from build123d import *

# Parameters (mm, degrees)
SKETCH1_R           = 3.175
EXTRUSION2_DEPTH    = 6.35
SKETCH1_3_R         = 6.35
BOSS_EXTRUDE1_DEPTH = 6.35
SKETCH1_4_R         = 3.175
CUT_EXTRUDE1_DEPTH  = 6.35


with BuildPart() as part:
    # Sketch1 → Extrusion2 (new body)
    with BuildSketch(Plane.XY):
        with BuildLine():
            Line((0, 0), (19.05, 0))
            ThreePointArc((19.05, 0), (12.7, 6.35), (19.05, 12.7))
            Line((19.05, 12.7), (0, 12.7))
            ThreePointArc((0, 12.7), (-6.35, 6.35), (0, 0))
        make_face()
        with Locations((0, 6.35)):
            Circle(SKETCH1_R, mode=Mode.SUBTRACT)
    extrude(amount=EXTRUSION2_DEPTH)

    # Sketch1<3> → Boss-Extrude1 (add)
    with BuildSketch(Plane.XY):
        with Locations((19.05, 6.35)):
            Circle(SKETCH1_3_R)
    extrude(amount=BOSS_EXTRUDE1_DEPTH)

    # Sketch1<4> → Cut-Extrude1 (cut)
    with BuildSketch(Plane.XY):
        with Locations((19.05, 6.35)):
            Circle(SKETCH1_4_R)
    extrude(amount=CUT_EXTRUDE1_DEPTH, mode=Mode.SUBTRACT)


solid = part.part
Verification items for the finished model (mm, model axes). Give positions to 0.01 mm unless a question says otherwise; leave off trailing zeros. Write each loop counter-clockwise with the first axis right and the second up, starting at its lowest first coordinate (ties: lowest second). Pieces come first, ordered by that corner, then holes. Notation, with made-up numbers: M -22,-7.75 L 18,-7.75 A17 cw 18,21.25 Z; hole C 22.25,79.25 d10. An arc over 180 degrees is marked long. Write item = value, one per line.
(1) Sectioned sample at D-D (y = 1). Record the cut outline in (x, z).
Found:
outline = M -3.42,0 L 22.47,0 L 22.47,6.35 L -3.42,6.35 Z
(2) Sectioned sample at B-B (z = 2.25). Record the cut outline in (x, y) (3 decimals).
Found:
outline = M 0,0 L 19.05,0 A6.35 ccw 19.05,12.7 L 0,12.7 A6.35 ccw Z; hole C 0,6.35 d6.35; hole C 19.05,6.35 d6.35
(3) Go/stop test with flat-tipped pins: pin 1 Ø4 at (x, y) = (15, 7.5) entering from -Z; pin 2 Ø1.5 at (y, z) = (9.5, 1) entering from +X. Record where each tip stops, or that it passes through.
Found:
pin_1 = 0
pin_2 = 24.93
(4) Sectioned sample at A-A (y = 6.35). Record the cut outline in (x, z) (3 decimals), then the cut area to 3 significant figures.
Found:
outline = M -6.35,0 L -3.175,0 L -3.175,6.35 L -6.35,6.35 Z; M 3.175,0 L 15.875,0 L 15.875,6.35 L 3.175,6.35 Z; M 22.225,0 L 25.4,0 L 25.4,6.35 L 22.225,6.35 Z
area = 121 mm2
(5) Sectioned sample at C-C (x = 21.5). Record the cut outline in (y, z), then the cut area to 3 significant figures.
Found:
outline = M 0.49,0 L 4.33,0 L 4.33,6.35 L 0.49,6.35 Z; M 8.37,0 L 12.21,0 L 12.21,6.35 L 8.37,6.35 Z
area = 48.8 mm2
(6) Material ranges on line 1 (X direction, y = 7.25, z = 3.25); line 2 (Y direction, x = 0, z = 2.5) (3 decimals); line 3 (X direction, y = 7, z = 5.5), recorded low to high.
Found:
line_1 = -6.29 to -3.04, 3.04 to 16.01, 22.09 to 25.34
line_2 = 0 to 3.175, 9.525 to 12.7
line_3 = -6.32 to -3.11, 3.11 to 15.94, 22.16 to 25.37
(7) Draft check along X on faces 1 (the face through (10, 12.7, 3)), 2 (the face through (25.4, 6.2, 3.1)), 3 (the face through (15.88, 6.49, 3.13)), 4 (the face through (1.707, 9.027, 3.131)). Enter one of: released by +X, released by -X, zero draft, split by the parting line, or undercut.
Found:
face_1 = zero draft
face_2 = released by +X
face_3 = undercut
face_4 = undercut
